Autodesk Inventor part; units mm, degrees
ref_plane "YZ Plane" through (0, 0, 0) normal (1, 0, 0) x (0, 1, 0)
ref_plane "XZ Plane" through (0, 0, 0) normal (0, 1, 0) x (-1, 0, 0)
ref_plane "XY Plane" through (0, 0, 0) normal (0, 0, 1) x (1, 0, 0)
sketch "Esquisse1" plane through (0, 0, 0) normal (0, 0, 1) x (1, 0, 0)
  line L0 (-36.1898, 0) -> (37.2521, 0)
  line L1 (0, 12.5) -> (-44.5, 12.5)
  line L2 (-44.5, 12.5) -> (-44.5, 36.75)
  line L3 (-44.5, 36.75) -> (0, 42.75)
  line L4 (0, 42.75) -> (0, 12.5)
  point P0 (0, 0)
  dimension "d0" = 25
  dimension "d1" = 85.5
  dimension "d2" = 0
  dimension "d3" = 73.5
  dimension "d4" = 44.5
  dimension "d5" = 0
revolve "Révolution1" add sketch "Esquisse1" angle 360 about axis through (-36.1898, 0, 0) along (1, 0, 0)
sketch "Esquisse3" plane through (0, 0, 0) normal (1, 0, 0) x (0, 0, -1)
  circle A0 centre (0, 0) radius 41
  circle A1 centre (0, 0) radius 12.5
  line L0 (0, 0) -> (-59.2945, 0)
  line L1 (0, 0) -> (0, -53.2291)
  line L2 (0, 0) -> (55.0659, 0)
  point P0 (0, -41)
  point P1 (41, 0)
  point P2 (-41, 0)
  dimension "d16" = 82
hole "Perçage1" at (0, -41, 0) at (0, 0, 41) at (0, 0, -41) direction (-1, 0, 0) diameter 10.106 depth 32.3 tip angle 118
sketch "Esquisse4" plane through (0, 0, 0) normal (1, 0, 0) x (0, 0, 1)
  line L0 (0, 0) -> (-39.036, -39.036)
  line L1 (0, 0) -> (-55.3193, 0)
  circle A0 centre (0, 0) radius 12.5
  line L2 (-5.5456, -11.2025) -> (-7.8791, -13.5359)
  line L3 (-11.2025, -5.5456) -> (-13.5359, -7.8791)
  line L4 (-13.5359, -7.8791) -> (-7.8791, -13.5359)
  dimension "d17" = 45
  dimension "d20" = 3.3
  dimension "d21" = 3.3
  dimension "d22" = 4
  dimension "d23" = 4
extrude "Extrusion1" cut sketch "Esquisse4" against normal through all contours A0 L2 L4 L0 | L0 L4 L3 A0
sketch "Esquisse5" plane through (0, 0, 0) normal (1, 0, 0) x (0, 0, 1)
  line L0 (-1, 17.25) -> (1, 17.25)
  line L1 (1, 17.25) -> (1, -42.75)
  line L2 (1, -42.75) -> (-1, -42.75)
  line L3 (-1, -42.75) -> (-1, 17.25)
  line L4 (-1, 17.25) -> (1, -42.75) construction
  line L5 (1, 17.25) -> (-1, -42.75) construction
  arc A0 (-4.8326, 42.476) -> (4.8326, 42.476) centre (0, 0) ccw
  point P0 (0, -12.75)
  point P1 (42.6948, 2.1722)
  point P2 (-42.6948, 2.1722)
  point P3 (4.9266, -42.4652)
  point P4 (42.5102, -4.5219)
  dimension "d26" = 2
  dimension "d27" = 60
  dimension "d28" = 0
extrude "Extrusion2" cut sketch "Esquisse5" against normal through all
properties part number "Douille2517"
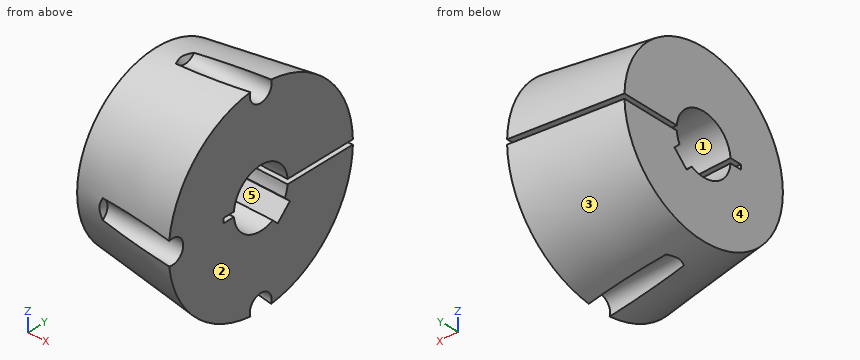
Work out the finished part from the listing and answer in its coordinate system (mm). Face numbers are marked on the shaded views. A direction names the side the tool comes from. Give positions to 0.01 mm unless a question says otherwise; leave off trailing zeros. Loops run counter-clockwise (first coordinate to the right, second up) from the corner with the lowest first, then second, coordinate; pieces in that order, holes last. Notation, with made-up numbers: (89.25, 52) - (99.25, 52) arc R24 cw to (99.25, 80) - close; hole circle Ø2 at (-25.75, -11.5). An arc over 180 degrees is marked (long way). Answer in a Markdown table with one row per item. Add a question column.
Q1. The part is cut by section C-C (x = -15). Determine the outline of the cut face in (y, z), and give its area (3 significant figures).
Q2. The part is cut by section B-B (x = -23.5). Determine the outline of the cut face in (y, z).
Q3. Determine the mould class of the marked faces 3, 4 and 5 for opening direction Y: released by +Y, released by -Y, zero draft, split by the parting line, or undercut.
Q4. Each of these flat-tipped pins is pushed along its axis until it touches: P1, Ø10, axis at x = -12, z = -18.5, coming from the -Y side; P2, Ø1.5, axis at x = -25, y = 2, coming from the +Z side; P3, Ø1.5, axis at x = -23.5, z = -31.5, coming from the -Y side. Where does it stop, or does it pass through?
Q5. A tool of negligible diameter and unlimited length cuts with its end or side. For the marked faces 1 and 2, from which of +Z, -Z, +X, -X, +Y, -Y can it reach the whole face along a straight path? Write none if from no direction.
Q6. The part is cut by section A-A (y = 0). Determine the outline of the cut face in (x, z).
Q7. Consider line 1 along Z through (x, y) = (-8, 0); line 2 along Z through (x, y) = (-37, -17); line 3 along Y through (x, z) = (-12.5, -7.5). Determine where each line is inside the solid, lowest interval first.
Solution:
| question | item | result |
|---|---|---|
| 1 | outline | (-40.42, -5.02) arc R40.73 ccw to (-5.02, -40.42) arc R5.05 cw to (5.02, -40.42) arc R40.73 ccw to (40.72, -1) - (12.46, -1) arc R12.5 cw to (11.2, -5.55) - (13.54, -7.88) - (7.88, -13.54) - (5.55, -11.2) arc R12.5 cw to (-12.46, -1) - (-17.25, -1) - (-17.25, 1) - (-12.46, 1) arc R12.5 cw to (12.46, 1) - (40.72, 1) arc R40.73 ccw to (5.02, 40.42) arc R5.05 cw to (-5.02, 40.42) arc R40.73 ccw to (-40.42, 5.02) arc R5.05 cw to start |
| 1 | area | 4,520 mm² |
| 2 | outline | (-39.29, -4.76) arc R39.58 ccw to (-4.76, -39.29) arc R5.05 cw to (4.76, -39.29) arc R39.58 ccw to (39.57, -1) - (12.46, -1) arc R12.5 cw to (11.2, -5.55) - (13.54, -7.88) - (7.88, -13.54) - (5.55, -11.2) arc R12.5 cw to (-12.46, -1) - (-17.25, -1) - (-17.25, 1) - (-12.46, 1) arc R12.5 cw to (12.46, 1) - (39.57, 1) arc R39.58 ccw to (4.76, 39.29) arc R5.05 cw to (-4.76, 39.29) arc R39.58 ccw to (-39.29, 4.76) arc R5.05 cw to start |
| 3 | face 3 | split by the parting line |
| 3 | face 4 | zero draft |
| 3 | face 5 | undercut |
| 4 | P1 | stops at y = -38.99 |
| 4 | P2 | stops at z = 36.76 |
| 4 | P3 | stops at y = -24.94 |
| 5 | face 1 | +X, -X |
| 5 | face 2 | +Z, -Z, +X, +Y, -Y |
| 6 | outline | (-44.5, -36.75) - (-33.66, -38.21) - (-32.3, -35.95) - (0, -35.95) - (0, -12.5) - (-44.5, -12.5) - close; (-44.5, 12.5) - (0, 12.5) - (0, 35.95) - (-32.3, 35.95) - (-33.66, 38.21) - (-44.5, 36.75) - close |
| 7 | line 1 | z = -35.95 to -12.5, 12.5 to 35.95 |
| 7 | line 2 | z = -33.72 to -1, 1 to 33.72 |
| 7 | line 3 | y = -40.37 to -10, 13.16 to 40.37 |
